The model under review builds one solid part; all positions refer to its coordinate system, in mm. Coordinates: 2 decimals unless noted, no trailing zeros. Write each loop counter-clockwise with the first axis right and the second up, starting at its lowest first coordinate (ties: lowest second). Pieces come first, ordered by that corner, then holes. Notation, with made-up numbers: (-8, 36.5) - (-1, 36.5) arc R10 ccw to (-1, 49.5) - close; hole circle Ø2 at (31, 30.25). An arc over 180 degrees is marked (long way). Put each result on its own line as item: value.
from build123d import *

# Parameters (mm, degrees)
SKETCH1_R                  = 15.1
SKETCH1_R_2                = 3
BOSS_EXTRUDE1_DEPTH        = 1.5
M1_6_CLEARANCE_HOLE2_D     = 1.8
M1_6_CLEARANCE_HOLE2_DEPTH = 11.5
CIRPATTERN1_COUNT          = 12
M1_6_CLEARANCE_HOLE1_D     = 1.8
M1_6_CLEARANCE_HOLE1_DEPTH = 11.5
CHAMFER2_SIZE              = 10.890667049
FILLET4_R                  = 5
CHAMFER3_SIZE              = 0.9
ESQUISSE1_R                = 0.9
ENL_V_MAT_EXTRU_1_DEPTH    = 71.229979354
CHANFREIN1_SIZE            = 0.9


with BuildPart() as part:
    # Sketch1 → Boss-Extrude1 (new body)
    with BuildSketch(Plane.XY):
        with BuildLine():
            Line((20.124611797, 6), (62.119198271, 4.998578975))
            ThreePointArc((62.119198271, 4.998578975), (67, 0), (62.119198271, -4.998578975))
            Line((62.119198271, -4.998578975), (20.124611797, -6))
            ThreePointArc((20.124611797, -6), (-21, 0), (20.124611797, 6))
        make_face()
        Circle(SKETCH1_R, mode=Mode.SUBTRACT)
        with Locations((46.5, 0)):
            Circle(SKETCH1_R_2, mode=Mode.SUBTRACT)
        with Locations((62, 0)):
            Circle(SKETCH1_R_2, mode=Mode.SUBTRACT)
    extrude(amount=BOSS_EXTRUDE1_DEPTH)

    # M1.6 Clearance Hole2
    with Locations(Plane.XY.offset(1.5)):
        with Locations((0, 17.5)):
            m1_6_clearance_hole2 = Hole(M1_6_CLEARANCE_HOLE2_D / 2, depth=M1_6_CLEARANCE_HOLE2_DEPTH)

    # CirPattern1: M1.6 Clearance Hole2 ×12 about axis
    cirpattern1_axis = Axis((0, 0, 0), (0, 0, 1))
    for i in range(1, CIRPATTERN1_COUNT):
        add(m1_6_clearance_hole2.rotate(cirpattern1_axis, i * 360 / CIRPATTERN1_COUNT), mode=Mode.SUBTRACT)

    # M1.6 Clearance Hole1
    with Locations(Plane.XY.offset(1.5)):
        with Locations((38.75, 2.5), (54.25, -2.5), (38.75, -2.5), (54.25, 2.5)):
            Hole(M1_6_CLEARANCE_HOLE1_D / 2, depth=M1_6_CLEARANCE_HOLE1_DEPTH)

    # Chamfer2
    # the kernel refuses this chamfer: 10.890667049, 7 mm, written as the material it adds along each edge
    with BuildSketch(Plane(origin=(20.124611797, -6, 0), x_dir=(-0.49038575496704445, -0.8715054855394783, 0), z_dir=(0, 0, 1))) as chamfer2_piece_1:
        with BuildLine():
            Line((9.279580073, 0), (-CHAMFER2_SIZE * 0.511022774248, CHAMFER2_SIZE * 0.85956717261))
            Line((-CHAMFER2_SIZE * 0.511022774248, CHAMFER2_SIZE * 0.85956717261), (0, 0))
            ThreePointArc((0, 0), (4.8297685, 0.518116548), (9.279580073, 0))
        make_face()
    extrude(amount=1.5)
    with BuildSketch(Plane(origin=(20.124611797, 6, 0), x_dir=(0.9997157950597969, -0.023839654107353114, 0), z_dir=(0, 0, 1))) as chamfer2_piece_2:
        with BuildLine():
            Line((CHAMFER2_SIZE, 0), (-4.742076753, 7.976422406))
            ThreePointArc((-4.742076753, 7.976422406), (-2.022765722, 4.41627981), (0, 0))
            Line((0, 0), (CHAMFER2_SIZE, 0))
        make_face()
    extrude(amount=1.5)

    # Fillet4
    fillet4_edges = [part.edges().sort_by_distance(p)[0] for p in [
        (31.012183665, -5.740370265, 0.75),
        (15.574037918, 14.087204937, 0.75),
        (15.574037918, -14.087204937, 0.75),
        (31.012183665, 5.740370265, 0.75),
    ]]
    fillet(fillet4_edges, radius=FILLET4_R)

    # Chamfer3
    chamfer3_edges = [part.edges().sort_by_distance(p)[0] for p in [
        (39.65, 2.5, 0),
        (55.15, 2.5, 0),
        (39.65, -2.5, 0),
        (55.15, -2.5, 0),
    ]]
    chamfer(chamfer3_edges, length=CHAMFER3_SIZE)

    # Esquisse1 → Enlèv. mat.-Extru.1 (cut, through all)
    with BuildSketch(Plane(origin=(0, 0, 0), x_dir=(-1, 0, 0), z_dir=(0, 0, -1))):
        with Locations((-25.251835753, 3.548914074)):
            Circle(ESQUISSE1_R)
        with Locations((-25.251835753, -3.548914074)):
            Circle(ESQUISSE1_R)
    extrude(amount=-ENL_V_MAT_EXTRU_1_DEPTH, mode=Mode.SUBTRACT)

    # Chanfrein1
    chanfrein1_edges = [part.edges().sort_by_distance(p)[0] for p in [
        (26.151835753, 3.548914074, 0),
        (26.151835753, -3.548914074, 0),
    ]]
    chamfer(chanfrein1_edges, length=CHANFREIN1_SIZE)


solid = part.part
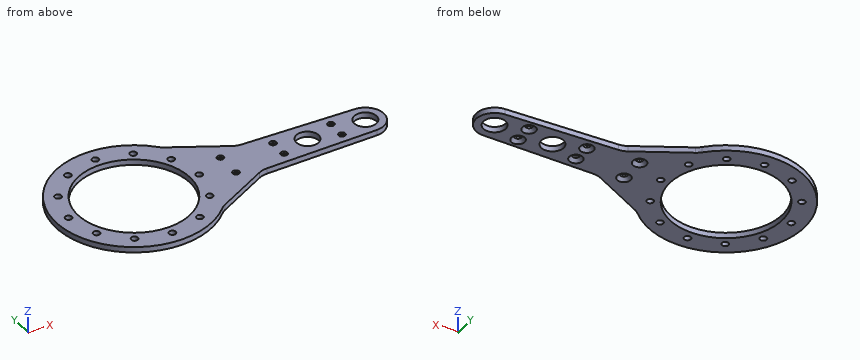
1. Consider section A-A on y = -17.5. State the section outline as (x, z) points, plus the area to 3 significant figures.
Determined:
outline: (-11.61, 0) - (-0.9, 0) - (-0.9, 1.5) - (-11.61, 1.5) - close; (0.9, 0) - (11.61, 0) - (11.61, 1.5) - (0.9, 1.5) - close
area: 32.1 mm^2
2. Consider section C-C on z = 0.4. Give the number of separate pieces and of enclosed holes in the cut face, plus the area to 3 significant figures.
Determined:
separate pieces: 1
enclosed holes: 21
area: 1,120 mm^2
3. For pin 1 Ø1.4 at (x, y) = (54.25, 2.5) entering from +Z; pin 2 Ø2 at (x, y) = (38.75, 2.5) entering from -Z, all flat-tipped, find the tip position at first contact; note any pin that passes through.
Determined:
pin 1: passes through
pin 2: stops at z = 0.8
4. Consider section D-D on x = 57. State the section outline as (y, z) points, plus the area to 3 significant figures.
Determined:
outline: (-5.12, 0) - (5.12, 0) - (5.12, 1.5) - (-5.12, 1.5) - close
area: 15.4 mm^2
5. Consider section B-B on x = 46.5. State the section outline as (y, z) points.
Determined:
outline: (-5.37, 0) - (-3, 0) - (-3, 1.5) - (-5.37, 1.5) - close; (3, 0) - (5.37, 0) - (5.37, 1.5) - (3, 1.5) - close
6. To check wall thickness, follow probe 1 along Y at (x, z) = (38.75, 1.15); probe 2 along Y at (x, z) = (8.5, 0.5); probe 3 along Y at (x, z) = (5.5, 1). State the ranges of each line that lie inside material, in increasing order.
Determined:
probe 1: y = -5.56 to -3.4, -1.6 to 1.6, 3.4 to 5.56
probe 2: y = -19.2 to -16.02, -14.29 to -12.48, 12.48 to 14.29, 16.02 to 19.2
probe 3: y = -20.27 to -14.06, 14.06 to 20.27
